Geometry: final body of the model. Coordinates: model frame, mm. A direction names the side the tool comes from. Give positions to 0.01 mm unless a question says otherwise; leave off trailing zeros. Write each loop counter-clockwise with the first axis right and the second up, starting at its lowest first coordinate (ties: lowest second). Pieces come first, ordered by that corner, then holes. Notation, with made-up numbers: (-4, 21.5) -> (19, 21.5) arc R18 cw to (19, 40.5) -> close; hole circle Ø8 at (-20, 47.5). An arc over 180 degrees is marked (long way). Answer as a JSON object with one key per item and string values.
Autodesk Inventor part; units mm, degrees
ref_plane "YZ Plane" through (0, 0, 0) normal (1, 0, 0) x (0, 1, 0)
ref_plane "XZ Plane" through (0, 0, 0) normal (0, 1, 0) x (-1, 0, 0)
ref_plane "XY Plane" through (0, 0, 0) normal (0, 0, 1) x (1, 0, 0)
sketch "Sketch1" plane through (0, 0, 0) normal (0, 1, 0) x (-1, 0, 0)
  point P0 (0, 0)
sketch "Sketch2" plane through (0, 0, 0) normal (0, 1, 0) x (-1, 0, 0)
  line L0 (0, 0) -> (177.8, 0)
  line L1 (177.8, 0) -> (177.8, -203.2)
  line L2 (0, 0) -> (0, -88.9)
  line L3 (177.8, -203.2) -> (107.95, -203.2)
  line L4 (107.95, -203.2) -> (107.95, -88.9)
  line L5 (0, -88.9) -> (107.95, -88.9)
  line L6 (190.5, -215.9) -> (190.5, 12.7)
  line L7 (190.5, 12.7) -> (-12.7, 12.7)
  line L8 (-12.7, 12.7) -> (-12.7, -101.6)
  line L9 (-12.7, -101.6) -> (95.25, -101.6)
  line L10 (95.25, -101.6) -> (95.25, -215.9)
  line L11 (95.25, -215.9) -> (190.5, -215.9)
  dimension "d0" = 203.2
  dimension "d1" = 177.8
  dimension "d2" = 88.9
  dimension "d3" = 69.85
  dimension "d4" = 12.7
extrude "Extrusion1" add sketch "Sketch2" along normal blind 6.35 contours L0 L1 L3 L4 L5 L2 | L11 L10 L9 L8 L7 L6
properties part number "RSX top" material "Aluminum 6061"
Q1. Cut plane C-C (x = -5.5). Return the cut outline in (y, z).
Values:
{"outline": "(0, -101.6) -> (6.35, -101.6) -> (6.35, 12.7) -> (0, 12.7) -> close"}
Q2. Material intervals for L1, parallel to Z at x = -14, y = 3.25; L2, parallel to X at y = 1, z = -133, sorted ascending. Write a range as from..to.
Values:
{"L1": "-101.6..12.7", "L2": "-190.5..-95.25"}
Q3. Set-up query: faces 1 (the flat face through (-110, 0, -75)), 2 (the flat face through (-95.25, 3, -158)). Return all of +Z, -Z, +X, -X, +Y, -Y with unobstructed straight access to the full face (end or side cutting, diameter ignored); none if empty.
Values:
{"face 1": "+Z, -Z, +X, -X, -Y", "face 2": "-Z, +X, +Y, -Y"}
Q4. Cut plane A-A (y = 1.5). Return the cut outline in (x, z), and give its area (3 significant figures).
Values:
{"outline": "(-190.5, -215.9) -> (-95.25, -215.9) -> (-95.25, -101.6) -> (12.7, -101.6) -> (12.7, 12.7) -> (-190.5, 12.7) -> close", "area": "34,100 mm²"}
Q5. First-contact query: P1, Ø3, axis at y = 2, z = -180.5, coming from the +X side; P2, Ø3, axis at x = -9.5, y = 4.5, coming from the -Z side. Flat tips, straight axial feed; report the tip coordinate or a pass-through.
Values:
{"P1": "x = -95.25", "P2": "z = -101.6"}
Q6. Cut plane B-B (z = -151). Return the cut outline in (x, y).
Values:
{"outline": "(-190.5, 0) -> (-95.25, 0) -> (-95.25, 6.35) -> (-190.5, 6.35) -> close"}
